```python
from build123d import *

# Parameters (mm, degrees)
F0_W     = 58.405198
F0_H     = 67.360154
F1_DEPTH = 76.2
F2_DEPTH = 12.7
F3_R     = 8.89
F4_R     = 3.81
F5_DEPTH = 25.4
F6_R     = 2.54
F7_DEPTH = 76.201
F6_R_2   = 5.08
F8_DEPTH = 2.54


with BuildPart() as f1:
    # F0 (on Front) → F1 (new body)
    with BuildSketch(Plane.XZ):
        Polygon((66.025198, -42.570077), (66.025198, 42.570077), (2.54, 42.570077), (-2.54, 42.570077), (-66.025198, 42.570077), (-66.025198, -42.570077), (-2.54, -42.570077), (2.54, -42.570077), align=None)
        with Locations((-31.742599, -3.81)):
            Rectangle(F0_W, F0_H, mode=Mode.SUBTRACT)
        with Locations((31.742599, -3.81)):
            Rectangle(F0_W, F0_H, mode=Mode.SUBTRACT)
    extrude(amount=F1_DEPTH)

    # F0 (on Front) → F2 (join)
    with BuildSketch(Plane.XZ):
        with Locations((-31.742599, -3.81)):
            Rectangle(F0_W, F0_H)
        with Locations((31.742599, -3.81)):
            Rectangle(F0_W, F0_H)
    extrude(amount=F2_DEPTH)

    # F3
    f3_edges = [f1.edges().sort_by_distance(p)[0] for p in [
        (66.025198, -38.1, 42.570077),
        (-66.025198, -38.1, -42.570077),
        (66.025198, -38.1, -42.570077),
        (-66.025198, -38.1, 42.570077),
    ]]
    fillet(f3_edges, radius=F3_R)

    # F4 (on face) → F5 (cut)
    with BuildSketch(Plane.XZ.offset(12.7)):
        with Locations((-34.964384, -0.660077)):
            Circle(F4_R)
        with Locations((34.385315, -0.660077)):
            Circle(F4_R)
    extrude(amount=-F5_DEPTH, mode=Mode.SUBTRACT)

    # F6 (on face) → F7 (cut, through all)
    with BuildSketch(Plane.XZ.offset(76.2)):
        with Locations((0, 36.728077)):
            Circle(F6_R)
    extrude(amount=-F7_DEPTH, mode=Mode.SUBTRACT)

    # F6 (on face) → F8 (join)
    with BuildSketch(Plane.XZ.offset(76.2)):
        with Locations((0, 36.728077)):
            Circle(F6_R_2)
        with Locations((0, 36.728077)):
            Circle(F6_R, mode=Mode.SUBTRACT)
    extrude(amount=F8_DEPTH)


solid = f1.part
```
Work out the finished part from the listing and answer in its coordinate system (mm). A direction names the side the tool comes from. Give positions to 0.01 mm unless a question says otherwise; leave off trailing zeros. Write each loop counter-clockwise with the first axis right and the second up, starting at its lowest first coordinate (ties: lowest second). Pieces come first, ordered by that corner, then holes. Notation, with made-up numbers: (77, 46.25) -> (122, 46.25) arc R16 cw to (122, 56.25) -> close; hole circle Ø6 at (86.25, 56.25). An arc over 180 degrees is marked (long way). Write each question's results on one line, items separated by ' | '.
1. Determine the mould class of faces 1 (the flat face through (31, -12.7, -3)), 2 (the flat face through (1, -38, 42.57)), 3 (the flat face through (66.025, -38, 0)) for opening direction Z: +Z half, -Z half, draft (parallel to the pull), parting line (faces both ways), or undercut.
Data:
face 1: undercut | face 2: +Z half | face 3: draft
2. This flat-tipped pin is pushed along its axis until it touches: pin 1 Ø12 at (x, z) = (-34.96, -0.66) entering from -Y. Where does it stop, or does it pass through?
Data:
pin 1: y = -12.7
3. Find section C-C on x = 53. Determine the outline of the cut face in (y, z).
Data:
outline: (-76.2, -42.57) -> (0, -42.57) -> (0, 42.57) -> (-76.2, 42.57) -> (-76.2, 29.87) -> (-12.7, 29.87) -> (-12.7, -37.49) -> (-76.2, -37.49) -> close
4. Find section B-B on z = -3. Determine the outline of the cut face in (x, y).
Data:
outline: (-66.03, -76.2) -> (-60.95, -76.2) -> (-60.95, -12.7) -> (-37.97, -12.7) -> (-37.97, 0) -> (-66.03, 0) -> close; (-31.96, -12.7) -> (-2.54, -12.7) -> (-2.54, -76.2) -> (2.54, -76.2) -> (2.54, -12.7) -> (31.38, -12.7) -> (31.38, 0) -> (-31.96, 0) -> close; (37.39, -12.7) -> (60.95, -12.7) -> (60.95, -76.2) -> (66.03, -76.2) -> (66.03, 0) -> (37.39, 0) -> close
5. A tool of negligible diameter and unlimited length cuts with its end or side. For faces 4 (the flat face through (-2.54, -44, -4)), 5 (the cylindrical face through (-63.352, -38.633, -40.035)), from which of +Z, -Z, +X, -X, +Y, -Y can it reach the whole face along a straight path? Write none if from no direction.
Data:
face 4: -Y | face 5: -Z, -X, +Y, -Y
6. Straight lines are drawn through the part: L1, parallel to X at y = -59, z = -4; L2, parallel to Z at x = -16.5, y = -57; L3, parallel to Z at x = 0, y = -48. For each, find the intervals that lie inside material, in ascending order.
Data:
L1: -66.03 to -60.95, -2.54 to 2.54, 60.95 to 66.03 | L2: -42.57 to -37.49, 29.87 to 42.57 | L3: -42.57 to 34.19, 39.27 to 42.57
7. Find section D-D on z = -19. Determine the outline of the cut face in (x, y), and give its area (3 significant figures).
Data:
outline: (-66.03, -76.2) -> (-60.95, -76.2) -> (-60.95, -12.7) -> (-2.54, -12.7) -> (-2.54, -76.2) -> (2.54, -76.2) -> (2.54, -12.7) -> (60.95, -12.7) -> (60.95, -76.2) -> (66.03, -76.2) -> (66.03, 0) -> (-66.03, 0) -> close | area: 2,640 mm^2
8. Find section A-A on x = 0. Determine the outline of the cut face in (y, z), and give its area (3 significant figures).
Data:
outline: (-78.74, 31.65) -> (-76.2, 31.65) -> (-76.2, -42.57) -> (0, -42.57) -> (0, 34.19) -> (-78.74, 34.19) -> close; (-78.74, 39.27) -> (0, 39.27) -> (0, 42.57) -> (-76.2, 42.57) -> (-76.2, 41.81) -> (-78.74, 41.81) -> close | area: 6,110 mm^2
